from build123d import *

# Parameters (mm, degrees)
BOSS_EXTRUDE1_DEPTH = 4.4
SKETCH2_W           = 10.6
SKETCH2_H           = 3.6
BOSS_EXTRUDE2_DEPTH = 3


with BuildPart() as part:
    # Sketch1 → Boss-Extrude1 (new body)
    with BuildSketch(Plane(origin=(0, 0, 0), x_dir=(0, 0, -1), z_dir=(1, 0, 0))):
        with BuildLine():
            Line((12.615293263, -92.633282396), (182.615293263, -92.633282396))
            ThreePointArc((182.615293263, -92.633282396), (98.271459614, -21.762843967), (84.825943994, 87.579368501))
            Line((84.825943994, 87.579368501), (131.929787104, 175.483372313))
            Line((131.929787104, 175.483372313), (210.884858569, 240.150484061))
            Line((210.884858569, 240.150484061), (308.236471933, 274.689971372))
            Line((308.236471933, 274.689971372), (415.1194685, 274.721469403))
            Line((415.1194685, 274.721469403), (612.615293263, 257.442823643))
            ThreePointArc((612.615293263, 257.442823643), (623.448797672, 266.533213196), (614.358408118, 277.366717604))
            Line((614.358408118, 277.366717604), (415.1194685, 294.797866154))
            Line((415.1194685, 294.797866154), (305.051694272, 294.797866154))
            Line((305.051694272, 294.797866154), (200.371020359, 260.785053385))
            Line((200.371020359, 260.785053385), (111.324320476, 196.088838941))
            Line((111.324320476, 196.088838941), (46.628106033, 107.042139058))
            Line((46.628106033, 107.042139058), (12.615293263, 2.361465145))
            Line((12.615293263, 2.361465145), (12.615293263, -92.633282396))
        make_face()
    extrude(amount=-BOSS_EXTRUDE1_DEPTH)

    # Sketch2 → Boss-Extrude2 (add)
    with BuildSketch(Plane.ZY.offset(4.4)):
        with BuildLine():
            Line((-614.358408118, 277.366717604), (-614.09694089, 274.37813351))
            Line((-614.09694089, 274.37813351), (-415.1194685, 291.786406641))
            Line((-415.1194685, 291.786406641), (-305.528662602, 291.786406641))
            Line((-305.528662602, 291.786406641), (-201.755236364, 258.068376511))
            Line((-201.755236364, 258.068376511), (-113.48028745, 193.932871967))
            Line((-113.48028745, 193.932871967), (-49.344782906, 105.657923053))
            Line((-49.344782906, 105.657923053), (-15.811778295, 2.453946809))
            Line((-15.811778295, 2.453946809), (-15.811778295, -92.633282396))
            Line((-15.811778295, -92.633282396), (-101.905821199, -92.633282396))
            Line((-101.905821199, -92.633282396), (-66.148126422, 3.910293146))
            Line((-66.148126422, 3.910293146), (-82.152924422, 88.94134))
            Line((-82.152924422, 88.94134), (-129.839029338, 177.574130079))
            Line((-129.839029338, 177.574130079), (-209.517623645, 242.833833686))
            Line((-209.517623645, 242.833833686), (-307.761340769, 277.689831483))
            Line((-307.761340769, 277.689831483), (-415.250010124, 277.721508004))
            Line((-415.250010124, 277.721508004), (-612.876760491, 260.431407737))
            Line((-612.876760491, 260.431407737), (-612.615293263, 257.442823643))
            ThreePointArc((-612.615293263, 257.442823643), (-623.448797672, 266.533213196), (-614.358408118, 277.366717604))
        make_face()
        with Locations((-40.615293263, -60.833282396)):
            Rectangle(SKETCH2_W, SKETCH2_H, mode=Mode.SUBTRACT)
        Polygon((-563.8078494, 273.256849808), (-553.2481856, 274.180700681), (-552.934424927, 270.594399768), (-563.494088726, 269.670548895), align=None, mode=Mode.SUBTRACT)
        Polygon((-473.552609753, 281.153160101), (-462.992945953, 282.077010974), (-462.679185279, 278.490710061), (-473.238849079, 277.566859188), align=None, mode=Mode.SUBTRACT)
        Polygon((-618.923562928, 268.735995644), (-608.363899128, 269.659846517), (-608.050138454, 266.073545604), (-618.609802254, 265.14969473), align=None, mode=Mode.SUBTRACT)
        Polygon((-62.703811589, -4.065338583), (-59.327925332, -5.315695323), (-63.009531289, -15.255804859), (-66.385417546, -14.005448119), align=None, mode=Mode.SUBTRACT)
    extrude(amount=BOSS_EXTRUDE2_DEPTH)


solid = part.part
CAD build for the part. Positions are in the model's coordinates, mm. A direction names the side the tool comes from. Round coordinates to 2 decimals unless told otherwise and drop trailing zeros. Loops run counter-clockwise (first coordinate to the right, second up) from the corner with the lowest first, then second, coordinate; pieces in that order, holes last. Notation, with made-up numbers: (34.5, 86) - (80.5, 86) arc R18 cw to (80.5, 117) - close; hole circle Ø10 at (81.5, 16). An arc over 180 degrees is marked (long way). Put each result on its own line as item: value.
1. Slice it at A-A on x = -2.75. List the corners of the cut face in (y, z).
Geometry check:
outline: (-92.63, -182.62) arc R150.46 cw to (87.58, -84.83) - (175.48, -131.93) - (240.15, -210.88) - (274.69, -308.24) - (274.72, -415.12) - (257.44, -612.62) arc R10 ccw to (277.37, -614.36) - (294.8, -415.12) - (294.8, -305.05) - (260.79, -200.37) - (196.09, -111.32) - (107.04, -46.63) - (2.36, -12.62) - (-92.63, -12.62) - close
2. Wall check: line 1 (Y direction, x = -5.5, z = -384.5); line 2 (Z direction, x = -6.5, y = 87); line 3 (Z direction, x = -2.25, y = -2). Give the ranges that are in metal, low to high.
Geometry check:
line 1: 277.71 to 291.79
line 2: -81.79 to -43.28
line 3: -89.33 to -12.62
3. Pin check, flat tips, straight feed: P1, Ø1.3, axis at x = -1.5, z = -355, coming from the -Y side; P2, Ø0.9, axis at x = -6, y = -61, coming from the -Z side; P3, Ø1.5, axis at x = -6, z = -337.5, coming from the -Y side. Stop position of each tip, or through.
Geometry check:
P1: y = 274.7
P2: z = -90.36
P3: y = 277.7
4. 3-axis set-ups, long thin cutter, end or side, ignore diameter. For faces 1 (the flat face through (-5.88, 282.96, -516)), 2 (the flat face through (-2.17, 130.92, -108.05)), 3 (the flat face through (-5.879, 54.778, -32.813)): which of +Z, -Z, +X, -X, +Y, -Y reach the whole face in a straight line?
Geometry check:
face 1: -X, +Y
face 2: -Z, +X, -X
face 3: +Z, -X, +Y
5. Slice it at C-C on z = -362. List the corners of the cut face in (x, y), and give its area (3 significant figures).
Geometry check:
outline: (-7.4, 277.71) - (-4.4, 277.71) - (-4.4, 274.71) - (0, 274.71) - (0, 294.8) - (-4.4, 294.8) - (-4.4, 291.79) - (-7.4, 291.79) - close
area: 131 mm²
6. Slice it at B-B on y = 69.5. List the corners of the cut face in (x, z).
Geometry check:
outline: (-7.4, -78.49) - (-4.4, -78.49) - (-4.4, -81.33) - (0, -81.33) - (0, -34.43) - (-4.4, -34.43) - (-4.4, -37.6) - (-7.4, -37.6) - close
7. Two-plate mould, pull along Z, no slides. Class faces 4 (the flat face through (-4.4, 39, -75)), 5 (the flat face through (-5.879, 269.197, -512.68)), 6 (the flat face through (-2.17, 152.19, -79.43)), 7 (the flat face through (-5.879, 132.637, -105.662)): released by +Z, released by -Z, zero draft, split by the parting line, or undercut.
Geometry check:
face 4: undercut
face 5: undercut
face 6: released by +Z
face 7: released by -Z
